Geometry check sheet. Reference: the model listing, model coordinates, mm. Face numbers are marked on the shaded views. A direction names the side the tool comes from. Coordinates: 2 decimals unless noted, no trailing zeros. Loops run counter-clockwise (first coordinate to the right, second up) from the corner with the lowest first, then second, coordinate; pieces in that order, holes last. Notation, with made-up numbers: (-16, -31) -> (32, -31) arc R16 ccw to (32, -2) -> close; hole circle Ø11 at (72, 75.5). An arc over 180 degrees is marked (long way). Answer as a JSON object with one key per item and string values.
from build123d import *

# Parameters (mm, degrees)
F1_DEPTH     = 55
F2_DEPTH     = 5
F3_DEPTH     = 15
F4_DEPTH     = 15
F5_R         = 2
F6_T1_DEPTH  = 14.1054111362
F6_T6_DEPTH  = 2
F6_T12_DEPTH = 171.8572508491
F7_R         = 2


# Not quite as in the source:
# - a fillet or chamfer that OpenCascade refuses, or shapes differently, is made with other operations: its cross-section is extruded or revolved along the edge and cut away or added
# - a feature names something its author has since deleted; it is built from what else it names


with BuildPart() as f1:
    # F0 (on Top) → F1 (new body)
    with BuildSketch(Plane.XY):
        with BuildLine():
            ThreePointArc((93, 77.5), (92.267766953, 79.267766953), (90.5, 80))
            Line((90.5, 80), (36.5, 80))
            Line((36.5, 80), (24.5, 80))
            Line((24.5, 80), (19, 80))
            Line((19, 80), (-7, 80))
            Line((-7, 80), (-12.5, 80))
            Line((-12.5, 80), (-24.5, 80))
            Line((-24.5, 80), (-74, 80))
            Line((-74, 80), (-91.5, 80))
            ThreePointArc((-91.5, 80), (-93.267766953, 79.267766953), (-94, 77.5))
            Line((-94, 77.5), (-94, 76))
            Line((-94, 76), (-94, 0))
            Line((-94, 0), (-94, -1.5))
            ThreePointArc((-94, -1.5), (-93.267766953, -3.267766953), (-91.5, -4))
            Line((-91.5, -4), (-88, -4))
            Line((-88, -4), (-73, -4))
            Line((-73, -4), (-28.6959191337, -4))
            Line((-28.6959191337, -4), (67.7072161436, -4))
            Line((67.7072161436, -4), (88, -4))
            Line((88, -4), (90.5, -4))
            ThreePointArc((90.5, -4), (92.267766953, -3.267766953), (93, -1.5))
            Line((93, -1.5), (93, 0))
            Line((93, 0), (93, 76))
            Line((93, 76), (93, 77.5))
        make_face()
        with BuildLine():
            ThreePointArc((90, 2.5), (89.267766953, 0.732233047), (87.5, 0))
            Line((87.5, 0), (-87.5, 0))
            ThreePointArc((-87.5, 0), (-89.267766953, 0.732233047), (-90, 2.5))
            Line((-90, 2.5), (-90, 73.5))
            ThreePointArc((-90, 73.5), (-89.267766953, 75.267766953), (-87.5, 76))
            Line((-87.5, 76), (87.5, 76))
            ThreePointArc((87.5, 76), (89.267766953, 75.267766953), (90, 73.5))
            Line((90, 73.5), (90, 2.5))
        make_face(mode=Mode.SUBTRACT)
    extrude(amount=F1_DEPTH)

    # F0 (on Top) → F2 (join)
    with BuildSketch(Plane.XY):
        with BuildLine():
            Line((-87.5, 0), (87.5, 0))
            ThreePointArc((87.5, 0), (89.267766953, 0.732233047), (90, 2.5))
            Line((90, 2.5), (90, 73.5))
            ThreePointArc((90, 73.5), (89.267766953, 75.267766953), (87.5, 76))
            Line((87.5, 76), (-87.5, 76))
            ThreePointArc((-87.5, 76), (-89.267766953, 75.267766953), (-90, 73.5))
            Line((-90, 73.5), (-90, 2.5))
            ThreePointArc((-90, 2.5), (-89.267766953, 0.732233047), (-87.5, 0))
        make_face()
        with BuildLine():
            Line((-77.5, 66), (77.5, 66))
            ThreePointArc((77.5, 66), (79.267766953, 65.267766953), (80, 63.5))
            Line((80, 63.5), (80, 12.5))
            ThreePointArc((80, 12.5), (79.267766953, 10.732233047), (77.5, 10))
            Line((77.5, 10), (-77.5, 10))
            ThreePointArc((-77.5, 10), (-79.267766953, 10.732233047), (-80, 12.5))
            Line((-80, 12.5), (-80, 63.5))
            ThreePointArc((-80, 63.5), (-79.267766953, 65.267766953), (-77.5, 66))
        make_face(mode=Mode.SUBTRACT)
        with BuildLine():
            Line((-24.5, 80), (-12.5, 80))
            Line((-12.5, 80), (-12.5, 89.5))
            ThreePointArc((-12.5, 89.5), (-13.232233047, 91.267766953), (-15, 92))
            Line((-15, 92), (-22, 92))
            ThreePointArc((-22, 92), (-23.767766953, 91.267766953), (-24.5, 89.5))
            Line((-24.5, 89.5), (-24.5, 80))
        make_face()
        with BuildLine():
            Line((-7, 80), (19, 80))
            Line((19, 80), (19, 89.5))
            ThreePointArc((19, 89.5), (18.267766953, 91.267766953), (16.5, 92))
            Line((16.5, 92), (-4.5, 92))
            ThreePointArc((-4.5, 92), (-6.267766953, 91.267766953), (-7, 89.5))
            Line((-7, 89.5), (-7, 80))
        make_face()
        with BuildLine():
            Line((24.5, 80), (36.5, 80))
            Line((36.5, 80), (36.5, 89.5))
            ThreePointArc((36.5, 89.5), (35.767766953, 91.267766953), (34, 92))
            Line((34, 92), (27, 92))
            ThreePointArc((27, 92), (25.232233047, 91.267766953), (24.5, 89.5))
            Line((24.5, 89.5), (24.5, 80))
        make_face()
    extrude(amount=F2_DEPTH)

    # F0 (on Top) → F3 (join)
    with BuildSketch(Plane.XY):
        with BuildLine():
            Line((93, -81.5), (93, -1.5))
            ThreePointArc((93, -1.5), (92.267766953, -3.267766953), (90.5, -4))
            Line((90.5, -4), (88, -4))
            Line((88, -4), (67.7072161436, -4))
            ThreePointArc((67.7072161436, -4), (74.7782839555, -6.9289321881), (77.7072161436, -14))
            Line((77.7072161436, -14), (77.7072161436, -58.7379819401))
            ThreePointArc((77.7072161436, -58.7379819401), (73.0879609173, -67.1669549309), (63.4976990076, -67.8088124137))
            Line((63.4976990076, -67.8088124137), (-32.9054362697, -23.0708304737))
            ThreePointArc((-32.9054362697, -23.0708304737), (-38.4608642113, -11.8445771571), (-28.6959191337, -4))
            Line((-28.6959191337, -4), (-73, -4))
            Line((-73, -4), (-73, -10.9733034172))
            Line((-73, -10.9733034172), (78.7072161436, -81.5))
            Line((78.7072161436, -81.5), (93, -81.5))
        make_face()
    extrude(amount=F3_DEPTH)

    # F0 (on Top) → F4 (join)
    with BuildSketch(Plane.XY):
        Polygon((-88, -4), (-73, -10.9733034172), (-73, -4), align=None)
        Polygon((-73, -34), (-73, -10.9733034172), (-88, -4), (-88, -34), align=None)
    extrude(amount=F4_DEPTH)

    # F5
    f5_edges = [f1.edges().sort_by_distance(p)[0] for p in [
        (85.853608, -81.5, 15),
    ]]
    fillet(f5_edges, radius=F5_R)

    # F6: fillet of radius 2 on 1 edges, made by hand

    # F6_s2 → F6_t1 (cut)
    with BuildSketch(Plane.XY.offset(-1.1054111362)):
        with BuildLine():
            ThreePointArc((78.3062611352, -81.3136012713), (78.7176414075, -81.4528444053), (79.1493805981, -81.5))
            Line((79.1493805981, -81.5), (78.7072161436, -81.5))
            Line((78.7072161436, -81.5), (78.3062611352, -81.3136012713))
        make_face()
    extrude(amount=F6_T1_DEPTH, mode=Mode.SUBTRACT)


with BuildPart() as f6_tool4:
    # F6_s5 → F6_t6 (new body)
    with BuildSketch(Plane.XY.offset(13)):
        Polygon((79.1493805981, -79.5), (78.3062611352, -81.3136012713), (78.7072161436, -81.5), (79.1493805981, -81.5), align=None)
    extrude(amount=F6_T6_DEPTH)

    # F6_s7 → F6_t8 (revolve, cut)
    with BuildSketch(Plane(origin=(79.1493805981, -79.5, 13), x_dir=(0.2158695953, 0.9764222027, 0), z_dir=(0.9764222027, -0.2158695953, 0))):
        with BuildLine():
            ThreePointArc((0, -2), (2, 0), (0, 2))
            Line((0, 2), (0, -2))
        make_face()
    revolve(axis=Axis((79.1493805981, -79.5, 13), (0, 0, 1)), mode=Mode.SUBTRACT)


with BuildPart() as f1_1:
    add(f1.part)

    # F6_t3: cut F6_tool4
    add(f6_tool4.part, mode=Mode.SUBTRACT)


with BuildPart() as f6_tool10:
    # F6_s11 → F6_t12 (new body)
    with BuildSketch(Plane(origin=(-60.3662112187, 28.0634604648, 0), x_dir=(0, 0, 1), z_dir=(0.9068006357, -0.4215597314, 0))):
        with BuildLine():
            ThreePointArc((15, 38.724458908), (14.4142135624, 40.1386724704), (13, 40.724458908))
            Line((13, 40.724458908), (15, 40.724458908))
            Line((15, 40.724458908), (15, 38.724458908))
        make_face()
    extrude(amount=F6_T12_DEPTH)

    split(bisect_by=Plane.YZ.offset(-73), keep=Keep.TOP)


with BuildPart() as f1_2:
    add(f1_1.part)

    # F6_t9: cut F6_tool10
    add(f6_tool10.part, mode=Mode.SUBTRACT)

    # F7
    f7_edges = [f1_2.edges().sort_by_distance(p)[0] for p in [
        (-80.5, -34, 15),
    ]]
    fillet(f7_edges, radius=F7_R)


solid = f1_2.part
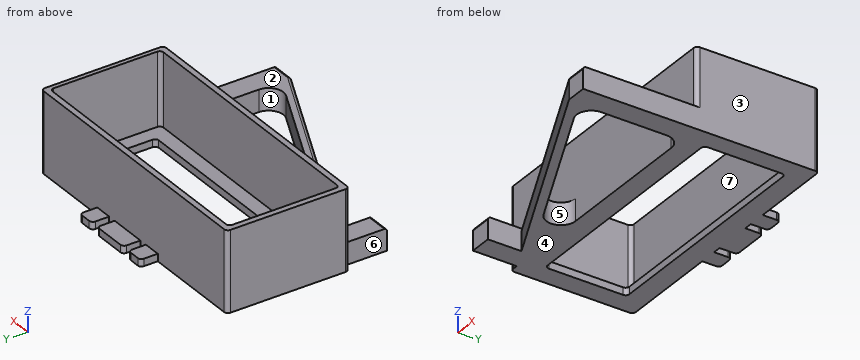
1. Section check A-A, the plane y = 41. Record the boundary of the cut face in (x, z), then the cut area to 3 significant figures.
Evaluation:
{"outline": "(-94, 0) -> (-80, 0) -> (-80, 5) -> (-90, 5) -> (-90, 55) -> (-94, 55) -> close; (80, 0) -> (93, 0) -> (93, 55) -> (90, 55) -> (90, 5) -> (80, 5) -> close", "area": "485 mm^2"}
2. Tool access check on the marked faces 4, 5, 6 and 7. Record the directions out of +Z, -Z, +X, -X, +Y, -Y that give a thin tool (end or side, any length) a straight path to the whole face; none if there is none.
Evaluation:
{"face 4": "-Z, +X, -X, +Y, -Y", "face 5": "+Z, -Z", "face 6": "+Z, -Z, -X, -Y", "face 7": "+Z"}
3. Thickness scan on probe 1 along Y at (x, z) = (-48, 40); probe 2 along X at (y, z) = (30, 13); probe 3 along Y at (x, z) = (25, 4.5). Record the ranges inside material, lowest first. Write a range as from..to.
Evaluation:
{"probe 1": "y = -4..0, 76..80", "probe 2": "x = -94..-90, 90..93", "probe 3": "y = -56.53..-49.94, -4..10, 66..91"}
4. Mould release check, pull along X, two halves, no side actions. Record for the marked faces 1, 2 and 3: released by +X, released by -X, zero draft, split by the parting line, or undercut.
Evaluation:
{"face 1": "undercut", "face 2": "zero draft", "face 3": "released by +X"}
5. Section check B-B, the plane z = 24. Record the boundary of the cut face in (x, y).
Evaluation:
{"outline": "(-94, -1.5) arc R2.5 ccw to (-91.5, -4) -> (90.5, -4) arc R2.5 ccw to (93, -1.5) -> (93, 77.5) arc R2.5 ccw to (90.5, 80) -> (-91.5, 80) arc R2.5 ccw to (-94, 77.5) -> close; hole (-90, 2.5) arc R2.5 ccw to (-87.5, 0) -> (87.5, 0) arc R2.5 ccw to (90, 2.5) -> (90, 73.5) arc R2.5 ccw to (87.5, 76) -> (-87.5, 76) arc R2.5 ccw to (-90, 73.5) -> close"}
6. Depth check by flat-ended pin: P1, Ø2.5, axis at y = 83, z = 2, coming from the +X side; P2, Ø4, axis at y = 84, z = 3.5, coming from the -X side; P3, Ø9.5, axis at x = -18.5, y = 89, coming from the +Z side; P4, Ø12, axis at y = -3, z = 24.5, coming from the -X side. Enter the tip coordinate at first touch or a pass-through.
Evaluation:
{"P1": "stops at x = 36.5", "P2": "stops at x = -24.5", "P3": "stops at z = 5", "P4": "stops at x = -94"}
7. Section check C-C, the plane y = -16.5. State how many separate pieces and enclosed holes the cut face has, then the cut area to 3 significant figures.
Evaluation:
{"separate pieces": "3", "enclosed holes": "0", "area": "793 mm^2"}
